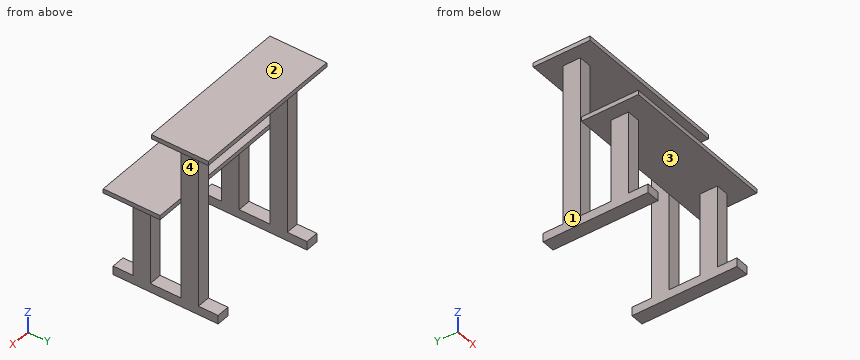
```python
from build123d import *

# Parameters (mm, degrees)
F0_W      = 914.4
F0_H      = 609.6
F1_DEPTH  = 1016
F2_W      = 914.4
F2_H      = 279.4
F3_DEPTH  = 457.2
F4_W      = 76.2
F4_H      = 609.6
F4_W_2    = 609.6
F5_DEPTH  = 533.4
F6_W      = 25.4
F6_H      = 431.8
F7_DEPTH  = 914.4
F8_W      = 76.2
F8_H      = 25.4
F8_W_2    = 609.6
F9_DEPTH  = 279.4
F8_H_2    = 431.8
F10_DEPTH = 431.8
F11_DEPTH = 330.2
F12_W     = 114.3
F12_H     = 939.8
F13_DEPTH = 777.24
F12_H_2   = 482.6
F14_DEPTH = 878.84


with BuildPart() as f1:
    # F0 (on Top) → F1 (new body)
    with BuildSketch(Plane.XY):
        Rectangle(F0_W, F0_H)
    extrude(amount=F1_DEPTH)

    # F2 (on face) → F3 (cut)
    with BuildSketch(Plane.XY.offset(1016)):
        with Locations((0, -165.1)):
            Rectangle(F2_W, F2_H)
    extrude(amount=-F3_DEPTH, mode=Mode.SUBTRACT)

    # F4 (on face) → F5 (cut)
    with BuildSketch(Plane(origin=(0, 0, 0), x_dir=(1, 0, 0), z_dir=(0, 0, -1))):
        with Locations((-419.1, 0)):
            Rectangle(F4_W, F4_H)
        with Locations((419.1, 0)):
            Rectangle(F4_W, F4_H)
        Rectangle(F4_W_2, F4_H)
    extrude(amount=-F5_DEPTH, mode=Mode.SUBTRACT)

    # F6 (on face) → F7 (cut)
    with BuildSketch(Plane(origin=(-457.2, 0, 0), x_dir=(0, -1, 0), z_dir=(-1, 0, 0))):
        with Locations((12.7, 774.7)):
            Rectangle(F6_W, F6_H)
    extrude(amount=-F7_DEPTH, mode=Mode.SUBTRACT)

    # F8 (on face) → F9 (cut)
    with BuildSketch(Plane(origin=(0, 304.8, 0), x_dir=(-1, 0, 0), z_dir=(0, 1, 0))):
        with Locations((-419.1, 546.1)):
            Rectangle(F8_W, F8_H)
        with Locations((0, 546.1)):
            Rectangle(F8_W_2, F8_H)
        with Locations((419.1, 546.1)):
            Rectangle(F8_W, F8_H)
    extrude(amount=-F9_DEPTH, mode=Mode.SUBTRACT)

    # F8 (on face) → F10 (cut)
    with BuildSketch(Plane(origin=(0, 304.8, 0), x_dir=(-1, 0, 0), z_dir=(0, 1, 0))):
        with Locations((0, 774.7)):
            Rectangle(F8_W_2, F8_H_2)
    extrude(amount=-F10_DEPTH, mode=Mode.SUBTRACT)

    # F8 (on face) → F11 (cut)
    with BuildSketch(Plane(origin=(0, 304.8, 0), x_dir=(-1, 0, 0), z_dir=(0, 1, 0))):
        with Locations((-419.1, 774.7)):
            Rectangle(F8_W, F8_H_2)
        with Locations((419.1, 774.7)):
            Rectangle(F8_W, F8_H_2)
    extrude(amount=-F11_DEPTH, mode=Mode.SUBTRACT)

    # F12 (on face) → F13 (cut)
    with BuildSketch(Plane(origin=(-381, 0, 0), x_dir=(0, -1, 0), z_dir=(-1, 0, 0))):
        with Locations((-247.65, 520.7)):
            Rectangle(F12_W, F12_H)
    extrude(amount=-F13_DEPTH, mode=Mode.SUBTRACT)

    # F12 (on face) → F14 (cut)
    with BuildSketch(Plane(origin=(-381, 0, 0), x_dir=(0, -1, 0), z_dir=(-1, 0, 0))):
        Polygon((0, 990.6), (-88.9, 990.6), (-88.9, 558.8), (-25.4, 558.8), (0, 558.8), align=None)
        Polygon((-88.9, 558.8), (-88.9, 50.8), (-25.4, 50.8), (-25.4, 533.4), (-25.4, 558.8), align=None)
        with Locations((31.75, 292.1)):
            Rectangle(F12_W, F12_H_2)
        with Locations((247.65, 292.1)):
            Rectangle(F12_W, F12_H_2)
    extrude(amount=-F14_DEPTH, mode=Mode.SUBTRACT)


solid = f1.part
```
Part model, mm, in its own coordinate system. Face numbers are marked on the shaded views. Round coordinates to 2 decimals unless told otherwise and drop trailing zeros. Order: outer loops, then holes, each group sorted by start corner. A loop starts at its lowest first (then second) coordinate and runs counter-clockwise, first axis right, second up. Notation, with made-up numbers: M -5.5,12.5 L 36.5,12.5 A10 ccw 36.5,18.5 Z; hole C 87,-19.75 d10. An arc over 180 degrees is marked long. Answer in a Markdown table with one row per item. Add a question column.
Q1. Wall check: L1, parallel to X at y = 58.5, z = 45; L2, parallel to Y at x = 331, z = 480.5; L3, parallel to Z at x = -107.5, y = 27.5. Give the ranges that are in metal, low to high. Write a range as from..to.
Q2. Cut at A-A on z = 726.5. Give the cut face in (x, y), and give its area (3 significant figures).
Q3. Mould opens along X. For the marked faces 1, 2, 3 and 4 say: +X half, -X half, draft (parallel to the pull), parting line (faces both ways), or undercut.
Q4. Cut at D-D on y = -162. Give the cut face in (x, z), and give its area (3 significant figures).
Q5. Cut at C-C on y = 220. Give the cut face in (x, z), and give its area (3 significant figures).
Q6. Pin check, flat tips, straight feed: pin 1 (23 mm diameter, centred on x = -345, y = -260.5, fed in from +Z); pin 2 (1.5 mm diameter, centred on x = -304.5, y = -2, fed in from -Z); pin 3 (8 mm diameter, centred on x = -251, y = -41.5, fed in from -Z); pin 4 (10 mm diameter, centred on x = 231.5, y = 87, fed in from -Z). Stop position of each tip, or through.
Q7. Cut at B-B on x = 263.5. Give the cut face in (y, z).
Established:
| question | item | result |
|---|---|---|
| 1 | L1 | x = -381..-304.8, 304.8..381 |
| 1 | L2 | y = -190.5..-88.9, 88.9..190.5 |
| 1 | L3 | z = 990.6..1016 |
| 2 | outline | M -381,88.9 L -304.8,88.9 L -304.8,190.5 L -381,190.5 Z; M 304.8,88.9 L 381,88.9 L 381,190.5 L 304.8,190.5 Z |
| 2 | area | 15,500 mm2 |
| 3 | face 1 | -X half |
| 3 | face 2 | draft |
| 3 | face 3 | undercut |
| 3 | face 4 | +X half |
| 4 | outline | M -457.2,533.4 L -381,533.4 L -381,0 L -304.8,0 L -304.8,533.4 L 304.8,533.4 L 304.8,0 L 381,0 L 381,533.4 L 457.2,533.4 L 457.2,558.8 L -457.2,558.8 Z |
| 4 | area | 105,000 mm2 |
| 5 | outline | M -457.2,990.6 L 457.2,990.6 L 457.2,1016 L -457.2,1016 Z; M -381,0 L -304.8,0 L -304.8,50.8 L -381,50.8 Z; M 304.8,0 L 381,0 L 381,50.8 L 304.8,50.8 Z |
| 5 | area | 31,000 mm2 |
| 6 | pin 1 | stops at z = 558.8 |
| 6 | pin 2 | stops at z = 0 |
| 6 | pin 3 | stops at z = 533.4 |
| 6 | pin 4 | stops at z = 990.6 |
| 7 | outline | M -304.8,533.4 L 25.4,533.4 L 25.4,558.8 L -304.8,558.8 Z; M -25.4,990.6 L 304.8,990.6 L 304.8,1016 L -25.4,1016 Z |
